Geometry: see drawing. Coordinates: mm, zero at the bounding-box minimum. A direction names the side the tool comes from. Round coordinates to 2 decimals unless told otherwise and drop trailing zeros. Order: outer loops, then holes, each group sorted by start corner. A loop starts at its lowest first (then second) coordinate and runs counter-clockwise, first axis right, second up. Notation, with made-up numbers: M 9.5,64 L 29.5,64 A24 cw 29.5,90 Z; hole C -1.75,53.5 d4. An arc over 180 degrees is marked long. Answer in a Markdown table with one row per item. Add a question column.
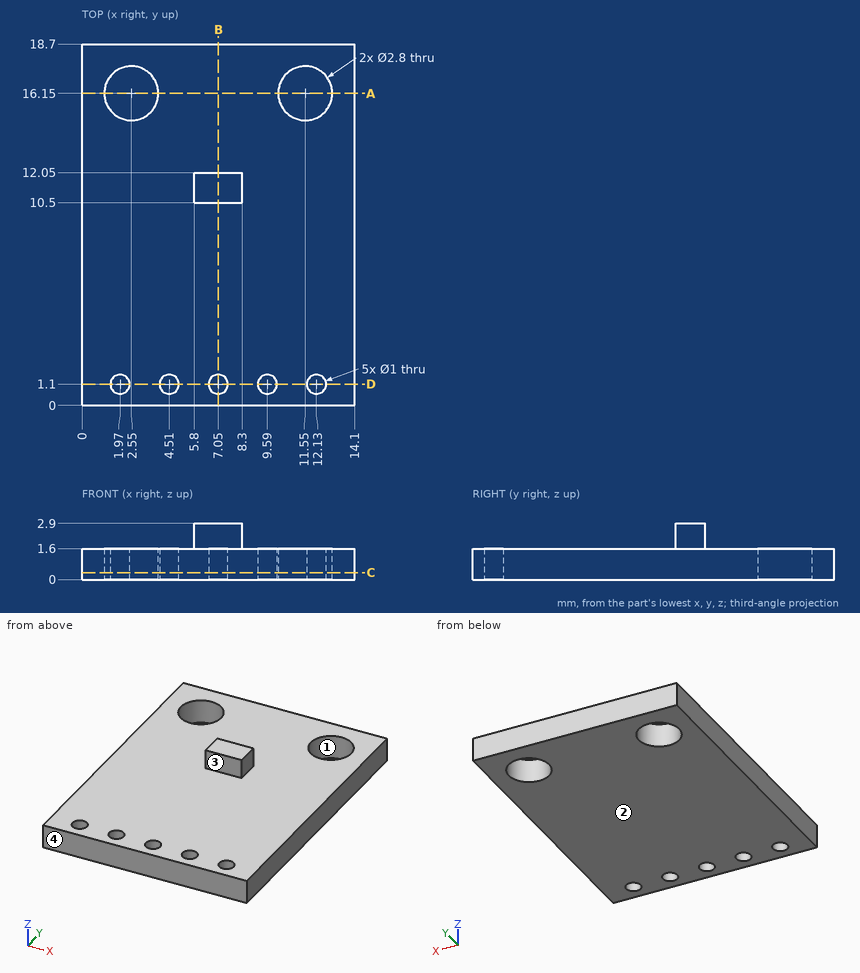
(1) Cut plane D-D (y = 1.1). Return loops of the section in (x, z).
(2) Access query for the marked faces 3 and 4. Directions: +Z, -Z, +X, -X, +Y, -Y. A direction counts if a zero-diameter tool reaches every point of the face in a straight line with its end or side. Return the directions, or none.
(3) Pin query (flat end, axial travel): pin 1 (2 mm diameter, centred on x = 4, y = 12, fed in from +Z); pin 2 (1 mm diameter, centred on x = 7.5, z = 2.5, fed in from +Y); pin 3 (0.7 mm diameter, centred on y = 11.5, z = 2, fed in from -X). Return the tip coordinate at first contact, or that it passes through.
(4) Cut plane A-A (y = 16.15). Return loops of the section in (x, z), and give its area (3 significant figures).
(5) Cut plane C-C (z = 0.35). Return loops of the section in (x, y).
(6) Draft query along X for the marked faces 1 and 2. Return one class per face: +X half, -X half, draft (parallel to the pull), parting line (faces both ways), or undercut.
(7) Line query: line 1 (Y direction, x = 2.55, z = 0.5); line 2 (Y direction, x = 9.59, z = 0.9); line 3 (Z direction, x = 5.25, y = 14.75). Output: solid intervals per line, ascending. Write a range as from..to.
(8) Cut plane B-B (x = 7.05). Return loops of the section in (y, z), and give its area (3 significant figures).
Answer list:
| question | item | result |
|---|---|---|
| 1 | outline | M 0,0 L 1.47,0 L 1.47,1.6 L 0,1.6 Z; M 2.47,0 L 4.01,0 L 4.01,1.6 L 2.47,1.6 Z; M 5.01,0 L 6.55,0 L 6.55,1.6 L 5.01,1.6 Z; M 7.55,0 L 9.09,0 L 9.09,1.6 L 7.55,1.6 Z; M 10.09,0 L 11.63,0 L 11.63,1.6 L 10.09,1.6 Z; M 12.63,0 L 14.1,0 L 14.1,1.6 L 12.63,1.6 Z |
| 2 | face 3 | +Z, +X, -X, -Y |
| 2 | face 4 | +Z, -Z, +X, -X, -Y |
| 3 | pin 1 | z = 1.6 |
| 3 | pin 2 | y = 12.05 |
| 3 | pin 3 | x = 5.8 |
| 4 | outline | M 0,0 L 1.15,0 L 1.15,1.6 L 0,1.6 Z; M 3.95,0 L 10.15,0 L 10.15,1.6 L 3.95,1.6 Z; M 12.95,0 L 14.1,0 L 14.1,1.6 L 12.95,1.6 Z |
| 4 | area | 13.6 mm² |
| 5 | outline | M 0,0 L 14.1,0 L 14.1,18.7 L 0,18.7 Z; hole C 2.55,16.15 d2.8; hole C 1.97,1.1 d1; hole C 4.51,1.1 d1; hole C 7.05,1.1 d1; hole C 9.59,1.1 d1; hole C 11.55,16.15 d2.8; hole C 12.13,1.1 d1 |
| 6 | face 1 | undercut |
| 6 | face 2 | draft |
| 7 | line 1 | 0..14.75, 17.55..18.7 |
| 7 | line 2 | 0..0.6, 1.6..18.7 |
| 7 | line 3 | 0..1.6 |
| 8 | outline | M 0,0 L 0.6,0 L 0.6,1.6 L 0,1.6 Z; M 1.6,0 L 18.7,0 L 18.7,1.6 L 12.05,1.6 L 12.05,2.9 L 10.5,2.9 L 10.5,1.6 L 1.6,1.6 Z |
| 8 | area | 30.3 mm² |
